The listing builds one solid part. Answer for the finished solid, in the listing's coordinates (mm). Face numbers are marked on the shaded views. A direction names the side the tool comes from. Round coordinates to 2 decimals unless told otherwise and drop trailing zeros. Order: outer loops, then holes, each group sorted by start corner. A loop starts at its lowest first (then second) coordinate and runs counter-clockwise, first axis right, second up. Notation, with made-up numbers: (85.25, -35.5) -> (133.25, -35.5) arc R21 ccw to (133.25, -24.5) -> close; hole circle Ø4 at (73, 57). An arc over 180 degrees is marked (long way). Return JSON: item names as keys, results as strings. Group by question number.
(1) The part is cut by section C-C (y = -5). Determine the outline of the cut face in (x, z), plus the area to 3 significant figures.
(2) Which of the six approach directions +Z, -Z, +X, -X, +Y, -Y give full straight-line access (tool end or side, diameter ignored) to the marked faces 1, 2 and 3?
(3) Consider line 1 (Y direction, x = 0, z = 3); line 2 (X direction, y = -20, z = 57); line 3 (Z direction, x = 15.5, y = -23.5). Determine where each line is inside the solid, lowest interval first. Write a range as [from, to].
(4) The part is cut by section B-B (z = 57.25). Determine the outline of the cut face in (x, y).
(5) The part is cut by section D-D (z = 22). Determine the outline of the cut face in (x, y).
(6) The part is cut by section A-A (x = 0). Determine the outline of the cut face in (y, z).
(7) Each of these flat-tipped pins is pushed along its axis until it touches: pin 1 (8 mm diameter, centred on x = 17, z = 27, fed in from -Y); pin 2 (4 mm diameter, centred on x = -11, y = -31.5, fed in from -Z); pin 3 (1.5 mm diameter, centred on y = -33.5, z = 17, fed in from -X); pin 4 (0.9 mm diameter, centred on x = -8.5, z = 3, fed in from -Y). Where does it stop, or does it pass through?
from build123d import *

# Parameters (mm, degrees)
F0_R      = 3.5
F1_DEPTH  = 9
F2_W      = 30
F2_H      = 8
F3_DEPTH  = 5
F5_DEPTH  = 60
F6_DEPTH  = 50
F7_DEPTH  = 9
F8_SIZE   = 7
F10_D     = 5
F10_DEPTH = 9
F10_TIP   = 1.5021515476
F11_W     = 7.2082555853
F11_H     = 16.9959962368
F12_DEPTH = 25
F13_R     = 1.5
F14_DEPTH = 33.001
F16_R     = 15.5
F17_DEPTH = 25


with BuildPart() as f1:
    # F0 (on Top) → F1 (new body)
    with BuildSketch(Plane.XY):
        with BuildLine():
            Line((-36, -7), (-36, -26))
            Line((-36, -26), (-32, -26))
            Line((-32, -26), (-32, -23))
            Line((-32, -23), (-31, -23))
            Line((-31, -23), (-3.6364618823, -44.4316388182))
            ThreePointArc((-3.6364618823, -44.4316388182), (0, -46), (3.6364618823, -44.4316388182))
            Line((3.6364618823, -44.4316388182), (26, -27.9666295471))
            Line((26, -27.9666295471), (36, -13))
            Line((36, -13), (36, -7))
            ThreePointArc((36, -7), (33.9497474683, -2.0502525317), (29, 0))
            Line((29, 0), (-29, 0))
            ThreePointArc((-29, 0), (-33.9497474683, -2.0502525317), (-36, -7))
        make_face()
        with Locations((0, -41)):
            Circle(F0_R, mode=Mode.SUBTRACT)
        with Locations((-29, -7)):
            Circle(F0_R, mode=Mode.SUBTRACT)
        with Locations((29, -7)):
            Circle(F0_R, mode=Mode.SUBTRACT)
    extrude(amount=F1_DEPTH)

    # F2 (on face) → F3 (cut)
    with BuildSketch(Plane.XY):
        with Locations((0, -19)):
            Rectangle(F2_W, F2_H)
    extrude(amount=F3_DEPTH, mode=Mode.SUBTRACT)

    # F4 (on face) → F5 (join)
    with BuildSketch(Plane.XY.offset(9)):
        Polygon((36, -13), (-36, -13), (-36, -23), (-32, -23), (-31, -23), (29.3184689522, -23), align=None)
    extrude(amount=F5_DEPTH)

    # F4 (on face) → F6 (join)
    with BuildSketch(Plane.XY.offset(9)):
        Polygon((39.8366187696, -21.6908202384), (36, -13), (29.3184689522, -23), (39, -23), align=None)
    extrude(amount=F6_DEPTH)

    # F4 (on face) → F7 (join)
    with BuildSketch(Plane.XY.offset(9)):
        Polygon((39.8366187696, -21.6908202384), (36, -13), (29.3184689522, -23), (39, -23), align=None)
    extrude(amount=-F7_DEPTH)

    # F8
    f8_edges = [f1.edges().sort_by_distance(p)[0] for p in [
        (39.418309, -22.34541, 0),
    ]]
    chamfer(f8_edges, length=F8_SIZE)

    # F10
    with Locations(Plane(origin=(25.3255301757, 11.1801189941, 0), x_dir=(-0.4038546073, 0.914823183, 0), z_dir=(0.914823183, 0.4038546073, 0))):
        with Locations((-30.9314672426, 16.5017858054), (-30.9314672426, 41.5017858054)):
            Hole(F10_D / 2, depth=F10_DEPTH)
            with Locations((0, 0, -(F10_DEPTH + F10_TIP / 2))):  # 118° drill point
                Cone(0, F10_D / 2, F10_TIP, mode=Mode.SUBTRACT)

    # F11 (on face) → F12 (join)
    with BuildSketch(Plane.XY.offset(9)):
        with Locations((0, -27.9626622796)):
            Rectangle(F11_W, F11_H)
    extrude(amount=F12_DEPTH)

    # F13 (on face) → F14 (cut, through all)
    with BuildSketch(Plane(origin=(0, -13, 0), x_dir=(-1, 0, 0), z_dir=(0, 1, 0))):
        with Locations((-6.9500040114, 2.750000149)):
            Circle(F13_R)
        with Locations((8.0499959886, 2.750000149)):
            Circle(F13_R)
        with Locations((8.0499959886, 57.250000149)):
            Circle(F13_R)
        with Locations((-6.9500040114, 57.250000149)):
            Circle(F13_R)
    extrude(amount=-F14_DEPTH, mode=Mode.SUBTRACT)

    # F16 (on face) → F17 (cut)
    with BuildSketch(Plane(origin=(0, -13, 0), x_dir=(-1, 0, 0), z_dir=(0, 1, 0))):
        with Locations((0, 35)):
            Circle(F16_R)
    extrude(amount=-F17_DEPTH, mode=Mode.SUBTRACT)


solid = f1.part
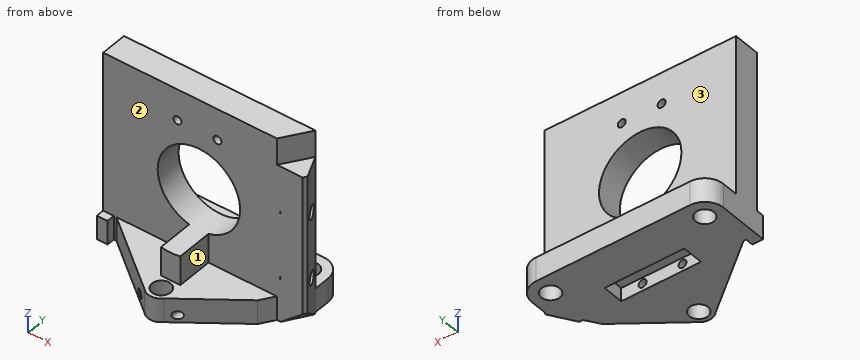
Answer below:
{
 "1": {"outline": "(-35.71, 0) -> (-31.87, 0) -> (-31.87, 9) -> (-35.71, 9) -> close; (-26.13, 0) -> (26.13, 0) -> (26.13, 9) -> (-26.13, 9) -> close; (31.87, 0) -> (35.71, 0) -> (35.71, 9) -> (31.87, 9) -> close", "area": "539 mm²"},
 "2": {"face 1": "+Z, +X, -Y", "face 2": "+Z, -Y", "face 3": "+Z, +X, -X, +Y"},
 "3": {"line 1": "y = [-46, -44.5], [-37.5, -23], [-15, 0]", "line 2": "x = [-36, -9.53], [-6.57, 5.47], [8.43, 39.09]", "line 3": "z = [0, 9]"},
 "4": {"outline": "(-36, -23) -> (-9.55, -23) -> (-9.55, -13) -> (-36, -13) -> close; (-6.55, -23) -> (5.45, -23) -> (5.45, -13) -> (-6.55, -13) -> close; (8.45, -23) -> (39, -23) -> (39.84, -21.69) -> (36, -13) -> (8.45, -13) -> close"},
 "5": {"outline": "(-36, -23) -> (-8.44, -23) -> (-8.44, -13) -> (-36, -13) -> close; (8.44, -23) -> (39, -23) -> (39.84, -21.69) -> (36, -13) -> (8.44, -13) -> close"},
 "6": {"outline": "(-46, 0) -> (-44.5, 0) -> (-44.5, 9) -> (-46, 9) -> close; (-37.5, 0) -> (-23, 0) -> (-23, 5) -> (-15, 5) -> (-15, 0) -> (0, 0) -> (0, 9) -> (-13, 9) -> (-13, 19.5) -> (-36.46, 19.5) -> (-36.46, 9) -> (-37.5, 9) -> close; (-23, 50.5) -> (-13, 50.5) -> (-13, 69) -> (-23, 69) -> close"},
 "7": {"pin 1": "stops at y = -23", "pin 2": "stops at z = 0", "pin 3": "stops at x = -3.6", "pin 4": "stops at y = -13"}
}
